```python
from build123d import *
from build123d.topology import SkipClean

# Parameters (mm, degrees)
SKETCH_1_W          = 13
SKETCH_1_H          = 29.5
EXTRUDE_1_DEPTH     = 7
EXTRUDE_2_DEPTH     = 4.5
SKETCH_3_W          = 7.2
SKETCH_3_H          = 7.2
SKETCH_3_R          = 2
EXTRUDE_3_DEPTH     = 2
CHAMFER_1_SIZE      = 1
CHAMFER_1_SIZE2     = 1.732050808
EXTRUDE_4_DEPTH     = 2
SKETCH_8_R          = 1.5
EXTRUDE_5_DEPTH     = 5.5
CUT_EXTRUDE_1_DEPTH = 35.949964235
SKETCH_10_R         = 3.7
CUT_EXTRUDE_2_DEPTH = 5.5
CUT_EXTRUDE_3_DEPTH = 3
CUT_EXTRUDE_4_DEPTH = 41.507530164
EXTRUDE_6_DEPTH     = 1
SKETCH_14_W         = 7.75
SKETCH_14_H         = 7.6
SKETCH_14_W_2       = 3.55
EXTRUDE_7_DEPTH     = 5


with BuildPart() as part:
    # Sketch 1 → Extrude 1 (new body)
    with BuildSketch(Plane(origin=(0, 0, 0), x_dir=(1, 0, 0), z_dir=(0, 1, 0))):
        with Locations((6.5, 14.75)):
            Rectangle(SKETCH_1_W, SKETCH_1_H)
    extrude_1 = extrude(amount=EXTRUDE_1_DEPTH)

    # Sketch 2 → Extrude 2 (add)
    with BuildSketch(Plane(origin=(0, 7, 0), x_dir=(1, 0, 0), z_dir=(0, 1, 0))):
        Polygon((6.5, 29.5), (10.75, 29.5), (10.75, 0), (2.25, 0), (2.25, 29.5), align=None)
    extrude(amount=EXTRUDE_2_DEPTH)

    # Sketch 5 → Cut-Revolve 2 (revolve, cut)
    with BuildSketch(Plane(origin=(6.5, 0, 0), x_dir=(0, 0, -1), z_dir=(1, 0, 0)), mode=Mode.PRIVATE) as cut_revolve_2_sk:
        with BuildLine():
            Line((29.5, 11.5), (24.5, 11.5))
            Line((24.5, 11.5), (24.5, 11.25))
            ThreePointArc((24.5, 11.25), (26.090990258, 10.590990258), (26.75, 9))
            Line((26.75, 9), (27, 9))
            Line((27, 9), (29.5, 11.5))
        make_face()
    revolve(cut_revolve_2_sk.sketch.rotate(Axis((6.5, 11.5, -24.5), (0, -1, 0)), 180), axis=Axis((6.5, 11.5, -24.5), (0, -1, 0)), mode=Mode.SUBTRACT)

    # Sketch 3 → Extrude 3 (add)
    # profile 1 of 3: a face of its own
    with BuildSketch(Plane(origin=(0, 11.5, 0), x_dir=(1, 0, 0), z_dir=(0, 1, 0))):
        with BuildLine():
            Line((3.4, 13.25), (3.4, 20.576990951))
            ThreePointArc((3.4, 20.576990951), (3.142346999, 20.795115883), (2.9, 21.030129685))
            Line((2.9, 21.030129685), (2.9, 12.75))
            Line((2.9, 12.75), (10.1, 12.75))
            Line((10.1, 12.75), (10.1, 21.030129685))
            ThreePointArc((10.1, 21.030129685), (9.857653001, 20.795115883), (9.6, 20.576990951))
            Line((9.6, 20.576990951), (9.6, 13.25))
            Line((9.6, 13.25), (3.4, 13.25))
        make_face()
    # profile 2 of 3: a face of its own
    with BuildSketch(Plane(origin=(0, 11.5, 0), x_dir=(1, 0, 0), z_dir=(0, 1, 0))):
        with BuildLine():
            Line((3.4, 20.576990951), (3.4, 20.75))
            Line((3.4, 20.75), (3.4, 28.25))
            Line((3.4, 28.25), (9.6, 28.25))
            Line((9.6, 28.25), (9.6, 20.576990951))
            ThreePointArc((9.6, 20.576990951), (9.857653001, 20.795115883), (10.1, 21.030129685))
            Line((10.1, 21.030129685), (10.1, 28.75))
            Line((10.1, 28.75), (6.5, 28.75))
            Line((6.5, 28.75), (2.9, 28.75))
            Line((2.9, 28.75), (2.9, 21.030129685))
            ThreePointArc((2.9, 21.030129685), (3.142346999, 20.795115883), (3.4, 20.576990951))
        make_face()
    # profile 3 of 3: a face of its own
    with BuildSketch(Plane(origin=(0, 11.5, 0), x_dir=(1, 0, 0), z_dir=(0, 1, 0))):
        with Locations((6.5, 4.35)):
            Rectangle(SKETCH_3_W, SKETCH_3_H)
        with Locations(Location((6.5, 4.35, 0), (0, 0, 270))):
            Circle(SKETCH_3_R, mode=Mode.SUBTRACT)
    extrude(amount=EXTRUDE_3_DEPTH)

    # Sketch 4 → Revolve 1 (revolve)
    with SkipClean():  # the faces are left unmerged after this step: merging them gives an invalid solid
        with BuildSketch(Plane(origin=(0, 11.5, 0), x_dir=(1, 0, 0), z_dir=(0, 1, 0))):
            with BuildLine():
                Line((4.5, 4.35), (6.5, 4.35))
                Line((6.5, 4.35), (8.5, 4.35))
                ThreePointArc((8.5, 4.35), (6.5, 6.35), (4.5, 4.35))
            make_face()
            with BuildLine():
                Line((8.5, 4.35), (6.5, 4.35))
                Line((6.5, 4.35), (4.5, 4.35))
                ThreePointArc((4.5, 4.35), (6.5, 2.35), (8.5, 4.35))
            make_face()
        revolve(axis=Axis((6.5, 11.5, -4.35), (1, 0, 0)))
    add(part.part.scale(1), mode=Mode.REPLACE)  # the faces are merged on a copy

    # Chamfer 1
    chamfer_1_edges = [part.edges().sort_by_distance(p)[0] for p in [
        (6.5, 13.5, -6.35),
    ]]
    chamfer_1_side = [part.faces().sort_by_distance(p)[0] for p in [
        (6.5, 13.5, -7.848176624),
    ]]
    chamfer(chamfer_1_edges, length=CHAMFER_1_SIZE, length2=CHAMFER_1_SIZE2, reference=chamfer_1_side[0])

    # Sketch 7 → Extrude 4 (add)
    with BuildSketch(Plane(origin=(0, 11.5, 0), x_dir=(1, 0, 0), z_dir=(0, 1, 0))):
        Polygon((2.25, 29.5), (10.75, 29.5), (10.75, 28.25), (10.75, 20.186921916), (9.6, 20.186921916), (9.6, 28.25), (3.4, 28.25), (3.4, 20.186921916), (2.25, 20.186921916), (2.25, 28.25), align=None)
    extrude(amount=-EXTRUDE_4_DEPTH)

    # Sketch 8 → Extrude 5 (add)
    with BuildSketch(Plane(origin=(0, 0, 0), x_dir=(-1, 0, 0), z_dir=(0, -1, 0))):
        with BuildLine():
            Line((-2.8, -3.7), (-2.8, 0))
            Line((-2.8, 0), (-10.2, 0))
            Line((-10.2, 0), (-10.2, -3.7))
            ThreePointArc((-10.2, -3.7), (-6.5, -7.4), (-2.8, -3.7))
        make_face()
        with Locations(Location((-6.5, -3.7, 0), (0, 0, 90))):
            Circle(SKETCH_8_R, mode=Mode.SUBTRACT)
    extrude_5 = extrude(amount=-EXTRUDE_5_DEPTH)

    # Sketch 9 → Cut-Extrude 1 (cut, through all)
    with BuildSketch(Plane.ZY):
        Polygon((10.785462846, 4.144098561), (7.4, 1.5), (1.9, 1.5), (1.9, 3), (0, 5.5), (7.4, 8.09796148), align=None)
    cut_extrude_1 = extrude(amount=-CUT_EXTRUDE_1_DEPTH, mode=Mode.SUBTRACT)

    # Sketch 10 → Cut-Extrude 2 (cut)
    with BuildSketch(Plane(origin=(0, 1.5, 0), x_dir=(1, 0, 0), z_dir=(0, 1, 0))):
        with Locations((6.5, -3.7)):
            Circle(SKETCH_10_R)
    cut_extrude_2 = extrude(amount=CUT_EXTRUDE_2_DEPTH, mode=Mode.SUBTRACT)

    # Mirror 1: Extrude 1, Extrude 5, Cut-Extrude 1, Cut-Extrude 2 across plane
    add(extrude_1.mirror(Plane(origin=(0, 0, -14.75), x_dir=(1, 0, 0), z_dir=(0, 0, -1))))
    add(extrude_5.mirror(Plane(origin=(0, 0, -14.75), x_dir=(1, 0, 0), z_dir=(0, 0, -1))))
    add(cut_extrude_1.mirror(Plane(origin=(0, 0, -14.75), x_dir=(1, 0, 0), z_dir=(0, 0, -1))), mode=Mode.SUBTRACT)
    add(cut_extrude_2.mirror(Plane(origin=(0, 0, -14.75), x_dir=(1, 0, 0), z_dir=(0, 0, -1))), mode=Mode.SUBTRACT)

    # Sketch 11 → Cut-Extrude 3 (cut)
    with BuildSketch(Plane(origin=(0, 0, 0), x_dir=(-1, 0, 0), z_dir=(0, -1, 0))):
        Polygon((-12.5, 9), (-12.5, 0.5), (-0.5, 0.5), (-0.5, 29), (-12.5, 29), (-12.5, 20.5), (-15.183114384, 20.5), (-15.183114384, 9), align=None)
    extrude(amount=-CUT_EXTRUDE_3_DEPTH, mode=Mode.SUBTRACT)

    # Sketch 12 → Cut-Extrude 4 (cut, through all)
    with BuildSketch(Plane(origin=(0, 3, 0), x_dir=(-1, 0, 0), z_dir=(0, -1, 0))):
        Polygon((-13, 20.5), (-13, 9), (-12.5, 9), (-10.75, 9), (-10.75, 20.5), (-12.5, 20.5), align=None)
    extrude(amount=-CUT_EXTRUDE_4_DEPTH, mode=Mode.SUBTRACT)

    # Sketch 13 → Extrude 6 (add)
    with BuildSketch(Plane(origin=(0, 3, 0), x_dir=(-1, 0, 0), z_dir=(0, -1, 0))):
        Polygon((-10.75, 9), (-10.75, 20.5), (-13, 20.5), (-18.5, 20.5), (-18.5, 9), align=None)
    extrude(amount=-EXTRUDE_6_DEPTH)

    # Sketch 14 → Extrude 7 (add)
    with BuildSketch(Plane(origin=(0, 4, 0), x_dir=(1, 0, 0), z_dir=(0, 1, 0))):
        with Locations((14.625, 14.75)):
            Rectangle(SKETCH_14_W, SKETCH_14_H)
        with Locations((20.275, 14.75)):
            Rectangle(SKETCH_14_W_2, SKETCH_14_H)
    extrude(amount=EXTRUDE_7_DEPTH)


solid = part.part
```
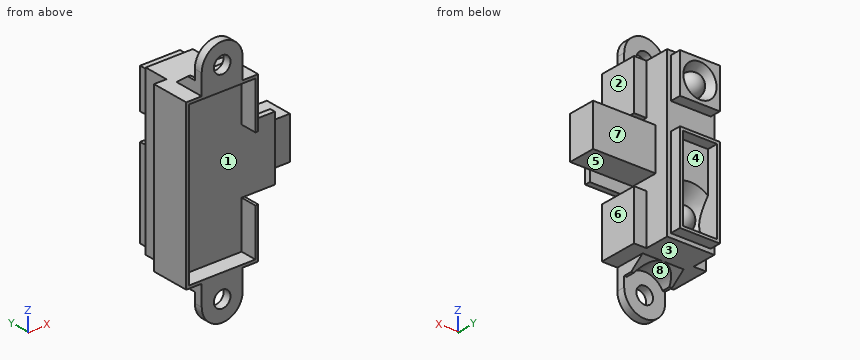
Verification items for the finished model (mm, model axes). Face numbers are marked on the shaded views. A direction names the side the tool comes from. Coordinates: 2 decimals unless noted, no trailing zeros. Loops run counter-clockwise (first coordinate to the right, second up) from the corner with the lowest first, then second, coordinate; pieces in that order, holes last. Notation, with made-up numbers: (-18.75, 35.25) -> (1.25, 35.25) arc R19 ccw to (1.25, 64.25) -> close; hole circle Ø7 at (-32, 65.5). An arc over 180 degrees is marked (long way). Answer in a Markdown table with one row per item. Add a question column.
1. Section check C-C, the plane z = -4.35. Enter the section's corners in (x, y), then the cut area to 3 significant figures.
2. Section check B-B, the plane x = 14. Enter the section's corners in (y, z), then the cut area to 3 significant figures.
3. Draft check along Z on the marked faces 1, 2 and 3. Enter one of: +Z half, -Z half, draft (parallel to the pull), parting line (faces both ways), or undercut.
4. Section check A-A, the plane y = 8. Enter the section's corners in (x, z).
5. Material ranges on probe 1 along X at (y, z) = (12.5, -20); probe 2 along X at (y, z) = (0.45, -33.2); probe 3 along X at (y, z) = (2.75, -16.5), recorded low to high. Write a range as [from, to].
6. Access from +Z, -Z, +X, -X, +Y, -Y to the whole of each face (thin tool, end or side, straight path). Record for the marked faces 4, 5, 6, 7 and 8.
7. Section check D-D, the plane y = 2.5. Enter the section's corners in (x, z).
8. Depth check by flat-ended pin: P1, Ø4, axis at x = 7, z = -19, coming from the -Y side; P2, Ø3.5, axis at x = 9, y = 6, coming from the -Z side; P3, Ø3, axis at x = 19, y = 9.5, coming from the -Z side. Enter the tip coordinate at first touch or a pass-through.
Derived:
| question | item | result |
|---|---|---|
| 1 | outline | (0, 0) -> (0.5, 0) -> (0.5, 3) -> (12.5, 3) -> (12.5, 0) -> (13, 0) -> (13, 7) -> (10.75, 7) -> (10.75, 11.5) -> (10.1, 11.5) -> (10.1, 13.5) -> (9.5, 13.5) -> (8.5, 11.77) -> (8.5, 11.5) arc R2 ccw to (4.5, 11.5) -> (4.5, 11.77) -> (3.5, 13.5) -> (2.9, 13.5) -> (2.9, 11.5) -> (2.25, 11.5) -> (2.25, 7) -> (0, 7) -> close |
| 1 | area | 104 mm² |
| 2 | outline | (3, -20.5) -> (4, -20.5) -> (4, -18.55) -> (9, -18.55) -> (9, -10.95) -> (4, -10.95) -> (4, -9) -> (3, -9) -> close |
| 2 | area | 49.5 mm² |
| 3 | face 1 | undercut |
| 3 | face 2 | draft |
| 3 | face 3 | -Z half |
| 4 | outline | (2.25, -29.5) -> (10.75, -29.5) -> (10.75, -18.55) -> (22.05, -18.55) -> (22.05, -10.95) -> (10.75, -10.95) -> (10.75, 0) -> (2.25, 0) -> close |
| 5 | probe 1 | x = [2.9, 3.4], [9.6, 10.1] |
| 5 | probe 2 | x = [2.8, 5], [8, 10.2] |
| 5 | probe 3 | x = [0, 0.5] |
| 6 | face 4 | +Y |
| 6 | face 5 | +X, +Y |
| 6 | face 6 | -Z, +X, +Y, -Y |
| 6 | face 7 | +Z, -Z, +X, +Y |
| 6 | face 8 | -Z, +Y |
| 7 | outline | (0, -29.5) -> (2.8, -29.5) -> (2.8, -31.4) -> (3.27, -31.4) arc R3.7 cw to (9.73, -31.4) -> (10.2, -31.4) -> (10.2, -29.5) -> (13, -29.5) -> (13, -20.5) -> (12.5, -20.5) -> (12.5, -29) -> (0.5, -29) -> (0.5, -0.5) -> (12.5, -0.5) -> (12.5, -9) -> (13, -9) -> (13, 0) -> (10.2, 0) -> (10.2, 1.9) -> (9.73, 1.9) arc R3.7 cw to (3.27, 1.9) -> (2.8, 1.9) -> (2.8, 0) -> (0, 0) -> close |
| 8 | P1 | stops at y = 3 |
| 8 | P2 | stops at z = -30.45 |
| 8 | P3 | stops at z = -18.55 |
